Here's how the part is built. I have some questions about the finished solid (model axes, mm). A direction names the side the tool comes from. Round coordinates to 2 decimals unless told otherwise and drop trailing zeros. Write each loop counter-clockwise with the first axis right and the second up, starting at its lowest first coordinate (ties: lowest second). Pieces come first, ordered by that corner, then holes. Notation, with made-up numbers: (17, 33.25) - (24, 33.25) arc R25 ccw to (24, 55.25) - close; hole circle Ø9 at (2.5, -12.5). An arc over 180 degrees is marked (long way). Use one line per item in the form item = value. Start each with the question number.
1. I want a section at C-C, the plane x = 114.3. List the corners of the cut face in (y, z) for me (3 decimals).
2. I want a section at B-B, the plane y = 0. State how many separate pieces and enclosed holes the cut face has, plus the area to 3 significant figures.
3. I want a section at D-D, the plane x = 44.45. List the corners of the cut face in (y, z) for me (3 decimals), plus the area to 3 significant figures.
4. If I drill on line 1 along Y through (x, z) = (114.3, 2.4); line 2 along Y through (x, z) = (44.45, 2.55); line 3 along X through (y, z) = (42, 4.1), over which ranges is the centre line in solid material (lowest first)?
5. We'd pull the mould along Y, two halves only. Please class faces 4 (the flat face through (43, 1, 4.445)), 5 (the cylindrical face through (102.114, -45.815, 2.254)), 6 (the cylindrical face through (-5.679, 56.867, 2.191)), 7 (the cylindrical face through (61.734, 23.811, 2.254)): +Y half, -Y half, draft (parallel to the pull), parting line (faces both ways), or undercut.
6. I want a section at A-A, the plane x = 0. List the corners of the cut face in (y, z) for me (3 decimals), plus the area to 3 significant figures.
7. Which directions (+Z, -Z, +X, -X, +Y, -Y) give clear straight access to the entire face, cutting with the end or side of a thin tool? Please do faces 1 (the cylindrical face through (109.234, 23.811, 2.254)), 2 (the cylindrical face through (-57.147, -0.569, 2.191)), 3 (the flat face through (79.27, -47.615, 2.191)).
8. Will these pins go through, and if not, where does the flat tip stop? pin 1 (1.3 mm diameter, centred on x = 116, z = 2.5, fed in from +Y); pin 2 (15 mm diameter, centred on x = 114.3, y = 42.6, fed in from +Z) (3 decimals); pin 3 (2 mm diameter, centred on y = -13, z = 1, fed in from -X); pin 4 (7.5 mm diameter, centred on x = 0, y = 45, fed in from +Z).
Autodesk Inventor part; units mm, degrees
ref_plane "YZ Plane" through (0, 0, 0) normal (1, 0, 0) x (0, 1, 0)
ref_plane "XZ Plane" through (0, 0, 0) normal (0, 1, 0) x (-1, 0, 0)
ref_plane "XY Plane" through (0, 0, 0) normal (0, 0, 1) x (1, 0, 0)
sketch "Boceto1" plane through (0, 0, 0) normal (0, 0, 1) x (1, 0, 0)
  circle A0 centre (0, 0) radius 57.15
  circle A1 centre (101.6, 0) radius 44.45
  circle A2 centre (-31.75, 47.519) radius 11.1125
  circle A3 centre (-31.75, -47.519) radius 11.1125
  circle A4 centre (114.3, 42.5971) radius 11.1125
  circle A5 centre (114.3, -42.5971) radius 11.1125
  line L0 (7.1437, 56.7018) -> (107.1562, 44.1014)
  circle A6 centre (44.45, 52.0016) radius 11.1125
  line L1 (7.1437, -56.7018) -> (107.1562, -44.1014)
  circle A7 centre (44.45, -52.0016) radius 11.1125
  dimension "d0" = 114.3
  dimension "d1" = 88.9
  dimension "d2" = 203.2
  dimension "d3" = 22.225
  dimension "d4" = 22.225
  dimension "d7" = 22.225
  dimension "d8" = 22.225
  dimension "d11" = 22.225
  dimension "d13" = 0
  dimension "d14" = 22.225
  dimension "d27" = 12.7
  dimension "d28" = 12.7
  dimension "d29" = 44.45
  dimension "d30" = 44.45
  dimension "d31" = 31.75
  dimension "d32" = 31.75
extrude "Extrusión1" add sketch "Boceto1" along normal blind 4.445
sketch "Boceto2" plane through (0, 0, 4.445) normal (0, 0, 1) x (1, 0, 0)
  arc A0 (-21.9537, 52.7651) -> (-40.3458, 40.4764) centre (-31.75, 47.519) ccw
  circle A1 centre (-31.75, 47.519) radius 4.7625
  arc A2 (-40.3458, -40.4764) -> (-21.9537, -52.7651) centre (-31.75, -47.519) ccw
  circle A3 centre (-31.75, -47.519) radius 4.7625
  arc A4 (33.4247, -53.3907) -> (55.4753, -50.6125) centre (44.45, -52.0016) ccw
  circle A5 centre (44.45, -52.0016) radius 4.7625
  arc A6 (55.4753, 50.6125) -> (33.4247, 53.3907) centre (44.45, 52.0016) ccw
  circle A7 centre (44.45, 52.0016) radius 4.7625
  arc A8 (124.4689, 38.1158) -> (103.3657, 44.5789) centre (114.3, 42.5971) ccw
  circle A9 centre (114.3, 42.5971) radius 4.7625
  arc A10 (103.3657, -44.5789) -> (124.4689, -38.1158) centre (114.3, -42.5971) ccw
  circle A11 centre (114.3, -42.5971) radius 4.7625
  point P0 (0, 0)
  dimension "d18" = 9.525
  dimension "d19" = 9.525
  dimension "d20" = 9.525
  dimension "d21" = 9.525
  dimension "d22" = 9.525
  dimension "d23" = 9.525
extrude "Extrusión2" cut sketch "Boceto2" against normal up to surface (4.445 mm away)
fillet "Empalme1" radius 6.35 12 edges at (-21.9537, -52.7651, 2.2225) (-40.3458, -40.4764, 2.2225) (33.4247, -53.3907, 2.2225) (55.4753, -50.6125, 2.2225) (124.4689, -38.1158, 2.2225) (-40.3458, 40.4764, 2.2225) (-21.9537, 52.7651, 2.2225) (33.4247, 53.3907, 2.2225) (55.4753, 50.6125, 2.2225) (103.3657, 44.5789, 2.2225) (124.4689, 38.1158, 2.2225) (103.3657, -44.5789, 2.2225)
sketch "Boceto3" plane through (0, 0, 0) normal (0, 0, -1) x (-1, 0, 0)
  circle A0 centre (0, 0) radius 7.1437
  circle A1 centre (0, -45) radius 6.35
  circle A2 centre (0, 45) radius 6.35
  line L0 (0, -45) -> (0, 0)
  line L1 (0, 0) -> (0, 45)
  dimension "d33" = 14.2875
  dimension "d34" = 12.7
  dimension "d35" = 12.7
  dimension "d36" = 45
  dimension "d37" = 45
extrude "Extrusión3" cut sketch "Boceto3" against normal up to surface (4.445 mm away)
sketch "Boceto4" plane through (0, 0, 4.445) normal (0, 0, 1) x (1, 0, 0)
  circle A0 centre (93.4212, 0) radius 5.5563
  line L0 (65.4212, -28) -> (121.4212, -28)
  line L1 (121.4212, -28) -> (121.4212, 28)
  line L2 (121.4212, 28) -> (65.4212, 28)
  line L3 (65.4212, 28) -> (65.4212, -28)
  line L4 (69.6712, -23.75) -> (117.1712, -23.75)
  line L5 (117.1712, -23.75) -> (117.1712, 23.75)
  line L6 (117.1712, 23.75) -> (69.6712, 23.75)
  line L7 (69.6712, 23.75) -> (69.6712, -23.75)
  circle A1 centre (74.8306, -23.75) radius 2.7781
  circle A2 centre (112.0118, -23.75) radius 2.7781
  circle A3 centre (122.3306, -23.75) radius 2.7781
  circle A4 centre (64.5118, -23.75) radius 2.7781
  line L8 (64.5118, -26.5281) -> (74.8306, -26.5281)
  line L9 (64.5118, -20.9719) -> (74.8306, -20.9719)
  line L10 (112.0118, -26.5281) -> (122.3306, -26.5281)
  line L11 (122.3306, -20.9719) -> (112.0118, -20.9719)
  circle A5 centre (74.8306, 23.75) radius 2.7781
  circle A6 centre (64.5118, 23.75) radius 2.7781
  line L12 (64.5118, 20.9719) -> (74.8306, 20.9719)
  line L13 (64.5118, 26.5281) -> (74.8306, 26.5281)
  circle A7 centre (112.0118, 23.75) radius 2.7781
  circle A8 centre (122.3306, 23.75) radius 2.7781
  line L14 (112.0118, 20.9719) -> (122.3306, 20.9719)
  line L15 (112.0118, 26.5281) -> (122.3306, 26.5281)
  circle A9 centre (98.5806, 0) radius 5.5563
  circle A10 centre (88.2618, 0) radius 5.5563
  line L16 (98.5806, 5.5563) -> (88.2618, 5.5563)
  line L17 (98.5806, -5.5563) -> (88.2618, -5.5563)
  point P0 (0, 0)
  dimension "d40" = 11.1125
  dimension "d41" = 56
  dimension "d42" = 56
  dimension "d43" = 28
  dimension "d44" = 28
  dimension "d45" = 0
  dimension "d46" = 93.4212
  dimension "d47" = 47.5
  dimension "d48" = 47.5
  dimension "d49" = 23.75
  dimension "d50" = 23.75
  dimension "d57" = 5.5563
  dimension "d58" = 5.1594
  dimension "d59" = 5.5563
  dimension "d60" = 5.5563
  dimension "d61" = 5.1594
  dimension "d62" = 5.1594
  dimension "d63" = 5.5563
  dimension "d64" = 5.1594
  dimension "d65" = 0
  dimension "d66" = 5.5563
  dimension "d67" = 5.5563
  dimension "d68" = 5.1594
  dimension "d69" = 5.1594
  dimension "d70" = 0
  dimension "d71" = 5.5563
  dimension "d72" = 5.5563
  dimension "d73" = 5.1594
  dimension "d74" = 5.1594
  dimension "d75" = 0
  dimension "d78" = 11.1125
  dimension "d79" = 11.1125
  dimension "d80" = 5.1594
  dimension "d81" = 5.1594
extrude "Extrusión4" cut sketch "Boceto4" against normal up to next contours A0 A9 A10 | A0 A9 | A9 A10 A0 | A0 L16 A9 | A9 L17 A0 | A0 A10 A9 | A0 A10 L16 | A10 A9 | A9 A10 A0 | L17 A10 A0 | A0 A10 | L8 A4 L3 | L3 A4 L9 L7 L4 A1 L8 | L10 A2 L4 L5 L11 L1 A3 | L1 A3 L10 | A4 L3 | L3 A4 | A1 L4 | A3 L1 | L1 A3 | A2 L4 | A4 L9 L3 | L4 A1 | L4 L7 L9 A1 | L1 L11 A3 | A2 L11 L5 L4 | L4 A2 | L12 A6 L3 | L3 A6 L13 A5 L6 L7 L12 | L14 L5 L6 A7 L15 L1 A8 | L1 A8 L14 | A6 L3 | L3 A6 | L7 L6 A5 L12 | A8 L1 | L1 A8 | L14 A7 L6 L5 | A6 L13 L3 | A5 L6 | L1 L15 A8 | A7 L6 | A5 L6 | L6 A7
equation "\"d16\" = t"
equation "\"d18\" = Q"
equation "\"d19\" = Q"
equation "\"d20\" = Q"
equation "\"d21\" = Q"
equation "\"d22\" = Q"
equation "\"d23\" = Q"
equation "\"d33\" = DF"
equation "\"d34\" = NF"
equation "\"d35\" = NF"
equation "\"d40\" = DM"
equation "\"d41\" = AM"
equation "\"d42\" = AM"
equation "\"d43\" = 0.5 * AM"
equation "\"d44\" = 0.5 * AM"
equation "\"d47\" = BM"
equation "\"d48\" = BM"
equation "\"d49\" = 0.5 * BM"
equation "\"d50\" = 0.5 * BM"
equation "\"d57\" = NM"
equation "\"d59\" = NM"
equation "\"d60\" = NM"
equation "\"d63\" = NM"
equation "\"d66\" = NM"
equation "\"d67\" = NM"
equation "\"d71\" = NM"
equation "\"d72\" = NM"
equation "\"d78\" = DM"
equation "\"d79\" = DM"
equation "\"t\" = 4.445"
equation "\"Q\" = 9.525"
equation "\"DF\" = 14.2875"
equation "\"NF\" = 12.7"
equation "\"DM\" = 11.1125"
equation "\"NM\" = 5.55625"
equation "\"CM\" = 93.4212"
equation "\"AM\" = 56"
equation "\"BM\" = 47.5"
properties part number "SIDE REDUCTION PLATE I"
Model answer:
q1.outline = (-53.71, 0) - (-47.36, 0) - (-47.36, 4.445) - (-53.71, 4.445) - close; (-37.835, 0) - (-26.528, 0) - (-26.528, 4.445) - (-37.835, 4.445) - close; (-20.972, 0) - (20.972, 0) - (20.972, 4.445) - (-20.972, 4.445) - close; (26.528, 0) - (37.835, 0) - (37.835, 4.445) - (26.528, 4.445) - close; (47.36, 0) - (53.71, 0) - (53.71, 4.445) - (47.36, 4.445) - close
q2.separate_pieces = 3
q2.enclosed_holes = 0
q2.area = 744 mm2
q3.outline = (-63.114, 0) - (-56.764, 0) - (-56.764, 4.445) - (-63.114, 4.445) - close; (-47.239, 0) - (47.239, 0) - (47.239, 4.445) - (-47.239, 4.445) - close; (56.764, 0) - (63.114, 0) - (63.114, 4.445) - (56.764, 4.445) - close
q3.area = 476 mm2
q4.line_1 = -53.71 to -47.36, -37.83 to -26.53, -20.97 to 20.97, 26.53 to 37.83, 47.36 to 53.71
q4.line_2 = -63.11 to -56.76, -47.24 to 47.24, 56.76 to 63.11
q4.line_3 = -41.79 to -5.6, 5.6 to 109.58, 119.02 to 125.4
q5.face_4 = draft
q5.face_5 = -Y half
q5.face_6 = +Y half
q5.face_7 = undercut
q6.outline = (-57.15, 0) - (-51.35, 0) - (-51.35, 4.445) - (-57.15, 4.445) - close; (-38.65, 0) - (-7.144, 0) - (-7.144, 4.445) - (-38.65, 4.445) - close; (7.144, 0) - (38.65, 0) - (38.65, 4.445) - (7.144, 4.445) - close; (51.35, 0) - (57.15, 0) - (57.15, 4.445) - (51.35, 4.445) - close
q6.area = 332 mm2
q7.face_1 = +Z, -Z
q7.face_2 = +Z, -Z, -X
q7.face_3 = +Z, -Z, -Y
q8.pin_1 = 53.66
q8.pin_2 = 4.445
q8.pin_3 = -55.88
q8.pin_4 = through
